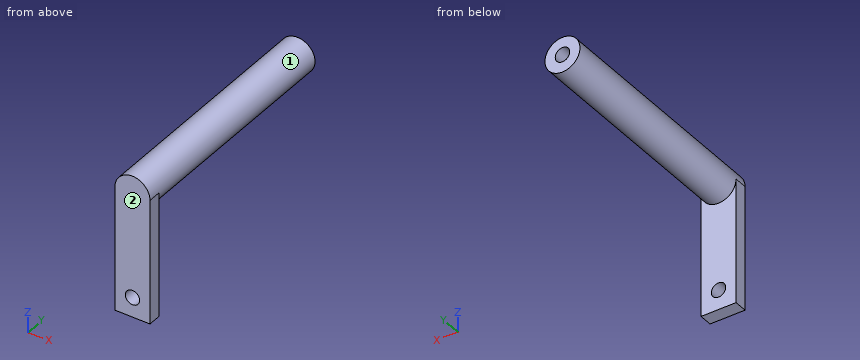
```python
from build123d import *

# Parameters (mm, degrees)
SKIZZE2_R                       = 1.65
SKIZZE2_R_2                     = 4
AUFSATZ_LINEAR_AUSTRAGEN1_DEPTH = 3
SKIZZE3_R                       = 4
AUFSATZ_LINEAR_AUSTRAGEN2_DEPTH = 52
SKIZZE4_R                       = 1.65
SCHNITT_LINEAR_AUSTRAGEN1_DEPTH = 10


with BuildPart() as part:
    # Skizze2 → Aufsatz-Linear austragen1 (new body)
    # profile 1 of 2: a face of its own
    with BuildSketch(Plane(origin=(0, 0, 0), x_dir=(1, 0, 0), z_dir=(0, 1, 0))):
        with BuildLine():
            Line((-4, 28.5), (-4, 0))
            ThreePointArc((-4, 0), (0, 4), (4, 0))
            Line((4, 0), (4, 28.5))
            Line((4, 28.5), (-4, 28.5))
        make_face()
        with Locations(Location((0, 24, 0), (0, 0, 270))):
            Circle(SKIZZE2_R, mode=Mode.SUBTRACT)
    # profile 2 of 2: a face of its own
    with BuildSketch(Plane(origin=(0, 0, 0), x_dir=(1, 0, 0), z_dir=(0, 1, 0))):
        Circle(SKIZZE2_R_2)
    extrude(amount=AUFSATZ_LINEAR_AUSTRAGEN1_DEPTH)

    # Skizze3 → Aufsatz-Linear austragen2 (add)
    with BuildSketch(Plane(origin=(0, 3, 0), x_dir=(1, 0, 0), z_dir=(0, 1, 0))):
        Circle(SKIZZE3_R)
    extrude(amount=AUFSATZ_LINEAR_AUSTRAGEN2_DEPTH)

    # Skizze4 → Schnitt-Linear austragen1 (cut)
    with BuildSketch(Plane(origin=(0, 55, 0), x_dir=(1, 0, 0), z_dir=(0, 1, 0))):
        with Locations(Location((0, 0, 0), (0, 0, 270))):
            Circle(SKIZZE4_R)
    extrude(amount=-SCHNITT_LINEAR_AUSTRAGEN1_DEPTH, mode=Mode.SUBTRACT)


solid = part.part
```
Input: part model. Units: mm. Frame: model coordinates. Face numbers are marked on the shaded views. A direction names the side the tool comes from. Give positions to 0.01 mm unless a question says otherwise; leave off trailing zeros. Write each loop counter-clockwise with the first axis right and the second up, starting at its lowest first coordinate (ties: lowest second). Pieces come first, ordered by that corner, then holes. Notation, with made-up numbers: (78.25, 85.5) - (100.25, 85.5) arc R19 ccw to (100.25, 91.5) - close; hole circle Ø10 at (-22.5, 58.5). An arc over 180 degrees is marked (long way). Write item = value, one per line. Start each with the question number.
1. Section query D-D, the plane x = 2.5. Output: boundary loops of the cut face in (y, z).
2. Section query C-C, the plane y = 48.5. Output: boundary loops of the cut face in (x, z), then the cut area to 3 significant figures.
3. Access query for the marked faces 1 and 2. Directions: +Z, -Z, +X, -X, +Y, -Y. A direction counts if a zero-diameter tool reaches every point of the face in a straight line with its end or side. Return the directions, or none.
4. Section query A-A, the plane z = -24. Output: boundary loops of the cut face in (x, y).
5. Section query B-B, the plane x = 0. Output: boundary loops of the cut face in (y, z), then the cut area to 3 significant figures.
6. Ray query, L1, parallel to X at y = 1.35, z = -24; L2, parallel to Y at x = -2.75, z = -27; L3, parallel to Z at x = 1, y = 30. Return the intervals inside material, ascending.
7. First-contact query: pin 1 Ø2 at (x, z) = (0.5, -9) entering from +Y; pin 2 Ø2 at (x, z) = (0, 0) entering from +Y. Flat tips, straight axial feed; report the tip coordinate or a pass-through.
Check sheet entries:
q1.outline = (0, -28.5) - (3, -28.5) - (3, -3.12) - (55, -3.12) - (55, 3.12) - (0, 3.12) - close
q2.outline = circle Ø8 at (0, 0); hole circle Ø3.3 at (0, 0)
q2.area = 41.7 mm2
q3.face_1 = +Y
q3.face_2 = +Z, -Z, +X, -X, -Y
q4.outline = (-4, 0) - (-1.65, 0) - (-1.65, 3) - (-4, 3) - close; (1.65, 0) - (4, 0) - (4, 3) - (1.65, 3) - close
q5.outline = (0, -28.5) - (3, -28.5) - (3, -25.65) - (0, -25.65) - close; (0, -22.35) - (3, -22.35) - (3, -4) - (55, -4) - (55, -1.65) - (45, -1.65) - (45, 1.65) - (55, 1.65) - (55, 4) - (0, 4) - close
q5.area = 471 mm2
q6.L1 = -4 to -1.65, 1.65 to 4
q6.L2 = 0 to 3
q6.L3 = -3.87 to 3.87
q7.pin_1 = 3
q7.pin_2 = 45
